Here's how the part is built. I have some questions about the finished solid (model axes, mm). Give positions to 0.01 mm unless a question says otherwise; leave off trailing zeros. Order: outer loops, then holes, each group sorted by start corner. A loop starts at its lowest first (then second) coordinate and runs counter-clockwise, first axis right, second up. Notation, with made-up numbers: M 57,22.5 L 76,22.5 A31 cw 76,60.5 Z; hole C 85.25,-23.5 d4. An arc over 180 degrees is marked long. One line per item, written item: value. Start each with the question number.
from build123d import *

# Parameters (mm, degrees)
F1_DEPTH     = 125
F2_R         = 175
F3_DEPTH     = 250
F4_R         = 124.99999
F5_T1_DEPTH  = 800
F5_T3_DEPTH  = 250
F5_T6_ANGLE  = 90
F5_T8_ANGLE  = 90
F5_T10_ANGLE = 90
F5_T12_ANGLE = 90
F5_T14_ANGLE = 90
F5_T16_ANGLE = 90
F5_T18_ANGLE = 90
F5_T20_ANGLE = 90
F5_T22_ANGLE = 180
F5_T24_ANGLE = 180
F6_R         = 175


# Not quite as in the source:
# - a fillet or chamfer that OpenCascade refuses, or shapes differently, is made with other operations: its cross-section is extruded or revolved along the edge and cut away or added
# - a fillet or chamfer is up to 0.001 mm smaller than in the source, because OpenCascade refuses the exact size


with BuildPart() as f1:
    # F0 (on Front) → F1 (new body, symmetric)
    with BuildSketch(Plane.XZ):
        with BuildLine():
            Line((400, -800), (400, 0))
            ThreePointArc((400, 0), (0, 400), (-400, 0))
            Line((-400, 0), (-400, -800))
            Line((-400, -800), (-150, -800))
            Line((-150, -800), (-150, -550))
            Line((-150, -550), (150, -550))
            Line((150, -550), (150, -800))
            Line((150, -800), (400, -800))
        make_face()
    extrude(amount=F1_DEPTH, both=True)

    # F2 (on face) → F3 (join, symmetric)
    with BuildSketch(Plane.XZ.offset(125)):
        Circle(F2_R)
    extrude(amount=F3_DEPTH, both=True)

    # F4 (radius 125 in the source; OpenCascade refuses exactly that, so slightly less here)
    f4_edges = [f1.edges().sort_by_distance(p)[0] for p in [
        (-400, 0, -800),
        (-275, 125, -800),
        (-150, 0, -800),
        (-275, -125, -800),
        (150, 0, -800),
        (275, 125, -800),
        (400, 0, -800),
        (275, -125, -800),
    ]]
    fillet(f4_edges, radius=F4_R)

    # F5: fillet of radius 125 on 8 edges, made by hand

    # F5_s2 → F5_t1 (cut)
    with BuildSketch(Plane.XY.offset(-800)):
        with BuildLine():
            ThreePointArc((275, -125), (363.3883476483, -88.3883476483), (400, 0))
            Line((400, 0), (400, -125))
            Line((400, -125), (275, -125))
        make_face()
        with BuildLine():
            ThreePointArc((275, 125), (363.3883476483, 88.3883476483), (400, 0))
            Line((400, 0), (400, 125))
            Line((400, 125), (275, 125))
        make_face()
        with BuildLine():
            ThreePointArc((-400, 0), (-363.3883476483, -88.3883476483), (-275, -125))
            Line((-275, -125), (-400, -125))
            Line((-400, -125), (-400, 0))
        make_face()
        with BuildLine():
            ThreePointArc((-400, 0), (-363.3883476483, 88.3883476483), (-275, 125))
            Line((-275, 125), (-400, 125))
            Line((-400, 125), (-400, 0))
        make_face()
    extrude(amount=F5_T1_DEPTH, mode=Mode.SUBTRACT)

    # F5_s4 → F5_t3 (cut)
    with BuildSketch(Plane.XY.offset(-800)):
        with BuildLine():
            ThreePointArc((-275, 125), (-186.6116523517, 88.3883476483), (-150, 0))
            Line((-150, 0), (-150, 125))
            Line((-150, 125), (-275, 125))
        make_face()
        with BuildLine():
            ThreePointArc((-275, -125), (-186.6116523517, -88.3883476483), (-150, 0))
            Line((-150, 0), (-150, -125))
            Line((-150, -125), (-275, -125))
        make_face()
        with BuildLine():
            ThreePointArc((275, -125), (186.6116523517, -88.3883476483), (150, 0))
            Line((150, 0), (150, -125))
            Line((150, -125), (275, -125))
        make_face()
        with BuildLine():
            ThreePointArc((275, 125), (186.6116523517, 88.3883476483), (150, 0))
            Line((150, 0), (150, 125))
            Line((150, 125), (275, 125))
        make_face()
    extrude(amount=F5_T3_DEPTH, mode=Mode.SUBTRACT)

    # F5_s5 → F5_t6 (revolve, cut)
    with BuildSketch(Plane.XZ):
        with BuildLine():
            ThreePointArc((274.99999, -800), (186.6116494227, -763.3883505773), (150, -675.00001))
            Line((150, -675.00001), (150, -800))
            Line((150, -800), (274.99999, -800))
        make_face()
    revolve(axis=Axis((275, 0, -800), (0, 0, -1)), revolution_arc=F5_T6_ANGLE, mode=Mode.SUBTRACT)

    # F5_s7 → F5_t8 (revolve, cut)
    with BuildSketch(Plane.YZ.offset(275)):
        with BuildLine():
            ThreePointArc((-1e-05, -800), (-88.3883505773, -763.3883505773), (-125, -675.00001))
            Line((-125, -675.00001), (-125, -800))
            Line((-125, -800), (-1e-05, -800))
        make_face()
    revolve(axis=Axis((275, 0, -800), (0, 0, -1)), revolution_arc=F5_T8_ANGLE, mode=Mode.SUBTRACT)

    # F5_s9 → F5_t10 (revolve, cut)
    with BuildSketch(Plane.XZ):
        with BuildLine():
            ThreePointArc((-274.99999, -800), (-186.6116494227, -763.3883505773), (-150, -675.00001))
            Line((-150, -675.00001), (-150, -800))
            Line((-150, -800), (-274.99999, -800))
        make_face()
    revolve(axis=Axis((-275, 0, -800), (0, 0, -1)), revolution_arc=F5_T10_ANGLE, mode=Mode.SUBTRACT)

    # F5_s11 → F5_t12 (revolve, cut)
    with BuildSketch(Plane.YZ.offset(-275)):
        with BuildLine():
            ThreePointArc((1e-05, -800), (88.3883505773, -763.3883505773), (125, -675.00001))
            Line((125, -675.00001), (125, -800))
            Line((125, -800), (1e-05, -800))
        make_face()
    revolve(axis=Axis((-275, 0, -800), (0, 0, -1)), revolution_arc=F5_T12_ANGLE, mode=Mode.SUBTRACT)

    # F5_s13 → F5_t14 (revolve, cut)
    with BuildSketch(Plane.XZ):
        with BuildLine():
            ThreePointArc((-275.00001, -800), (-363.3883505773, -763.3883505773), (-400, -675.00001))
            Line((-400, -675.00001), (-400, -800))
            Line((-400, -800), (-275.00001, -800))
        make_face()
    revolve(axis=Axis((-275, 0, -800), (0, 0, -1)), revolution_arc=F5_T14_ANGLE, mode=Mode.SUBTRACT)

    # F5_s15 → F5_t16 (revolve, cut)
    with BuildSketch(Plane.YZ.offset(-275)):
        with BuildLine():
            ThreePointArc((-1e-05, -800), (-88.3883505773, -763.3883505773), (-125, -675.00001))
            Line((-125, -675.00001), (-125, -800))
            Line((-125, -800), (-1e-05, -800))
        make_face()
    revolve(axis=Axis((-275, 0, -800), (0, 0, -1)), revolution_arc=F5_T16_ANGLE, mode=Mode.SUBTRACT)

    # F5_s17 → F5_t18 (revolve, cut)
    with BuildSketch(Plane.YZ.offset(275)):
        with BuildLine():
            ThreePointArc((1e-05, -800), (88.3883505773, -763.3883505773), (125, -675.00001))
            Line((125, -675.00001), (125, -800))
            Line((125, -800), (1e-05, -800))
        make_face()
    revolve(axis=Axis((275, 0, -800), (0, 0, -1)), revolution_arc=F5_T18_ANGLE, mode=Mode.SUBTRACT)

    # F5_s19 → F5_t20 (revolve, cut)
    with BuildSketch(Plane.XZ):
        with BuildLine():
            ThreePointArc((275.00001, -800), (363.3883505773, -763.3883505773), (400, -675.00001))
            Line((400, -675.00001), (400, -800))
            Line((400, -800), (275.00001, -800))
        make_face()
    revolve(axis=Axis((275, 0, -800), (0, 0, -1)), revolution_arc=F5_T20_ANGLE, mode=Mode.SUBTRACT)

    # F5_s21 → F5_t22 (revolve, cut)
    with BuildSketch(Plane.XY):
        with BuildLine():
            ThreePointArc((275, 125), (363.3883476483, 88.3883476483), (400, 0))
            Line((400, 0), (400, 125))
            Line((400, 125), (275, 125))
        make_face()
    revolve(axis=Axis((0, 125, 0), (0, -1, 0)), revolution_arc=F5_T22_ANGLE, mode=Mode.SUBTRACT)

    # F5_s23 → F5_t24 (revolve, cut)
    with BuildSketch(Plane.XY):
        with BuildLine():
            ThreePointArc((400, 0), (363.3883476483, -88.3883476483), (275, -125))
            Line((275, -125), (400, -125))
            Line((400, -125), (400, 0))
        make_face()
    revolve(axis=Axis((0, -125, 0), (0, -1, 0)), revolution_arc=F5_T24_ANGLE, mode=Mode.SUBTRACT)

    # F6
    f6_edges = [f1.edges().sort_by_distance(p)[0] for p in [
        (-175, -375, 0),
    ]]
    fillet(f6_edges, radius=F6_R)


solid = f1.part
Item 1: I want a section at C-C on y = -274. Write out the boundary of the cut face in (x, z).
Item 2: Please list where these lines run through material, in increasing order: probe 1 along X at (y, z) = (51.5, -611); probe 2 along Y at (x, z) = (-128, 163); probe 3 along X at (y, z) = (88.5, -620). Write a range as [from, to].
Item 3: Will these pins go through, and if not, where does the flat tip stop? P1, Ø6, axis at x = -252.5, z = 142.5, coming from the +Y side; P2, Ø10, axis at y = -162, z = -1, coming from the +X side; P3, Ø1.5, axis at x = 96.5, z = -508.5, coming from the -Y side.
Item 4: I want a section at D-D on z = -133. Write out the boundary of the cut face in (x, y).
Item 5: I want a section at A-A on z = -619. Write out the boundary of the cut face in (x, y), plus the area to 3 significant figures.
Item 6: We'd pull the mould along X, two halves only. Please class faces 1 (the face through (4, 2, -550)), 2 (the face through (-128.982, -163.025, 118.273)), 3 (the face through (-4, -125, -223)): +X half, -X half, draft (parallel to the pull), parting line (faces both ways), or undercut.
Item 7: I want a section at B-B on z = -371. Write out the boundary of the cut face in (x, y), plus the area to 3 significant figures.
Answer below:
1. outline: C 0,0 d317.17
2. probe 1: x = [-388.9, -161.1], [161.1, 388.9]
2. probe 2: y = [-125, 125]
2. probe 3: x = [-363.28, -186.72], [186.72, 363.28]
3. P1: stops at y = 124.43
3. P2: stops at x = 175
3. P3: stops at y = -125
4. outline: M -275,-125 L -113.74,-125 L -113.74,-200 A113.74 ccw 113.74,-200 L 113.74,-125 L 275,-125 A125 ccw 275,125 L -275,125 A125 ccw Z
5. outline: C -275,0 d250; C 275,0 d250
5. area: 98,200 mm²
6. face 1: undercut
6. face 2: parting line
6. face 3: draft
7. outline: M -275,-125 L 275,-125 A125 ccw 275,125 L -275,125 A125 ccw Z
7. area: 187,000 mm²
